from build123d import *

# Parameters (mm, degrees)
F0_R      = 2.675
F1_DEPTH  = 0.685
F1_FACE_R = 2.675
F3_R      = 1.5
F5_DEPTH  = 3.86
F7_R      = 1.2195
F5_FACE_R = 1.5
F9_DEPTH  = 1.1
F11_R     = 1


with BuildPart() as f1:
    # F0 (on Front) → F1 (new body)
    with BuildSketch(Plane.XZ):
        Circle(F0_R)
        Polygon((-1.1547005384, 0), (-0.5773502692, 1), (0.5773502692, 1), (1.1547005384, 0), (0.5773502692, -1), (-0.5773502692, -1), align=None, mode=Mode.SUBTRACT)
        Polygon((0.5773502692, 1), (-0.5773502692, 1), (-1.1547005384, 0), (-0.5773502692, -1), (0.5773502692, -1), (1.1547005384, 0), align=None)
    extrude(amount=-F1_DEPTH)

    # F1_face (on face) → F4 section 0
    with BuildSketch(Plane(origin=(0, 0.685, 0), x_dir=(1, 0, 0), z_dir=(0, 1, 0))):
        Circle(F1_FACE_R)
    # F3 (on offset) → F4 section 1
    with BuildSketch(Plane.XZ.offset(-1.175)):
        Circle(F3_R)
    loft()

    # F5 (add): a face of the model
    f5_faces = [f1.faces().sort_by_distance(p)[0] for p in [
        (0, 1.175, 0),
    ]]
    extrude(f5_faces, amount=F5_DEPTH)

    # F7 (on offset) → F8 section 0
    with BuildSketch(Plane(origin=(0, 5.315, 0), x_dir=(-1, 0, 0), z_dir=(0, 1, 0))):
        Circle(F7_R)
    # F5_face (on face) → F8 section 1
    with BuildSketch(Plane(origin=(0, 5.035, 0), x_dir=(-1, 0, 0), z_dir=(0, 1, 0))):
        Circle(F5_FACE_R)
    loft()

    # F0 (on Front) → F9 (cut)
    with BuildSketch(Plane.XZ):
        Polygon((0.5773502692, 1), (-0.5773502692, 1), (-1.1547005384, 0), (-0.5773502692, -1), (0.5773502692, -1), (1.1547005384, 0), align=None)
    extrude(amount=-F9_DEPTH, mode=Mode.SUBTRACT)

    # F11 (on offset) → F14 section 0
    with BuildSketch(Plane.XZ.offset(-1.1), mode=Mode.PRIVATE) as f14_s0:
        Circle(F11_R)
    loft([f14_s0.sketch, Vertex(0, 1.677, 0)], mode=Mode.SUBTRACT)


solid = f1.part
Build history of the part. All positions in model axes, mm. A direction names the side the tool comes from. Round coordinates to 2 decimals unless told otherwise and drop trailing zeros. Write each loop counter-clockwise with the first axis right and the second up, starting at its lowest first coordinate (ties: lowest second). Pieces come first, ordered by that corner, then holes. Notation, with made-up numbers: (10, 15) - (58, 15) arc R15 cw to (58, 35) - close; hole circle Ø6 at (-34.75, -26). An arc over 180 degrees is marked (long way). One line per question, with ' | ' between items.
1. Drill centre lines: line 1 along X through (y, z) = (1.15, -0.1); line 2 along Z through (x, y) = (0.55, 0.6); line 3 along Y through (x, z) = (-1.7, -1.45). Where is each one in solid material? Low to high. Write a range as from..to.
Results are:
line 1: -1.56..-0.91, 0.91..1.56 | line 2: -2.62..-1, 1..2.62 | line 3: 0..0.87
2. Drop flat-ended pins along their axis: pin 1 Ø0.5 at (x, z) = (-0.5, 0.5) entering from -Y; pin 2 Ø1 at (x, y) = (-1, 1) entering from +Z. Give the stop position or say it passes through.
Results are:
pin 1: y = 1.12 | pin 2: z = 2.6
3. Mould opens along X. For faces 1 (the face through (0, 0.5, -1)), 2 (the face through (0, 0, -1.2)), 3 (the face through (-0.035, 1.585, -0.156)), 4 (the face through (-0.58, 0.34, -2.61)) say: released by +X, released by -X, zero draft, split by the parting line, or undercut.
Results are:
face 1: undercut | face 2: zero draft | face 3: undercut | face 4: split by the parting line
4. Tool access for faces 5 (the face through (0.87, 0.54, 0.49)), 6 (the face through (-1.5, 3.08, 0.07)), 7 (the face through (0, 5.315, 0)): list every direction of +Z, -Z, +X, -X, +Y, -Y with a clear straight run to the whole face (end or side of a thin tool).
Results are:
face 5: -Y | face 6: +Y | face 7: +Z, -Z, +X, -X, +Y
5. Band-saw the part on A-A, the plane y = 3.6. Write the cut outline in (x, z), and give its area (3 significant figures).
Results are:
outline: circle Ø3 at (0, 0) | area: 7.07 mm^2
